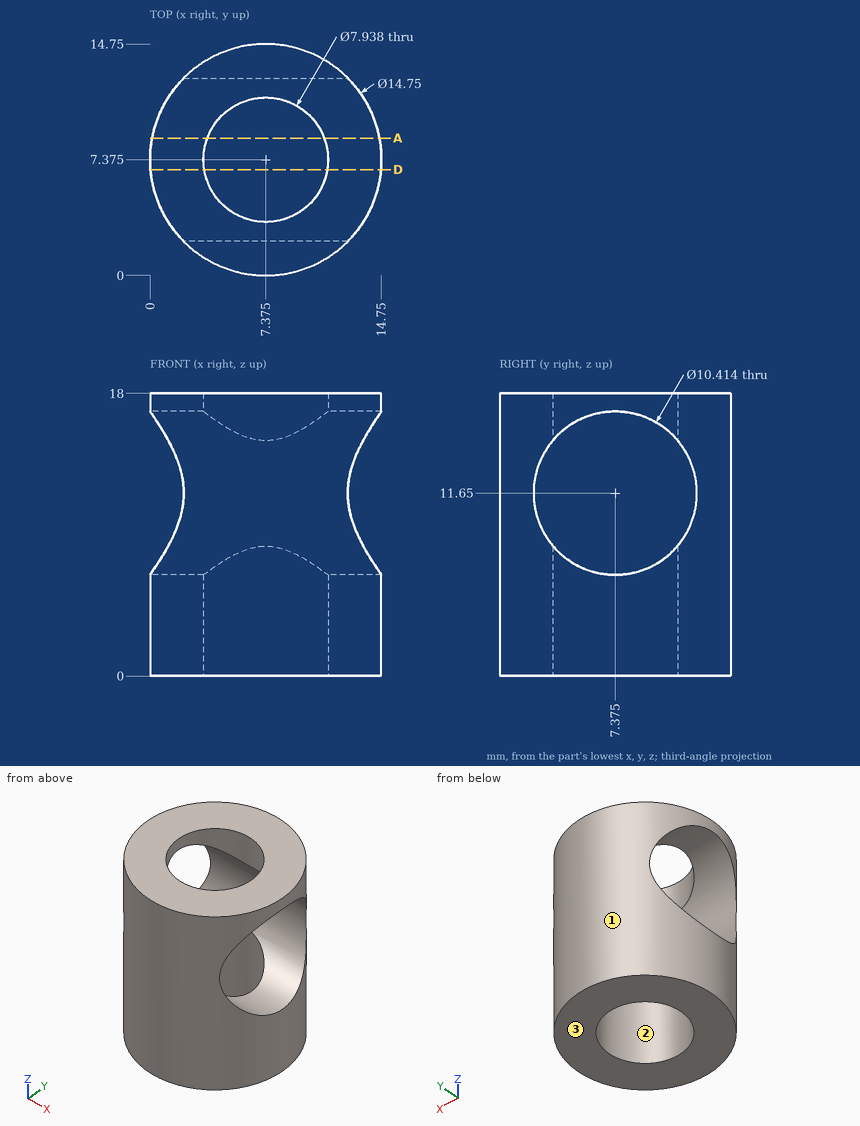
Geometry: see drawing. Coordinates: mm, zero at the bounding-box minimum. Give positions to 0.01 mm unless a question says otherwise; leave off trailing zeros. Order: outer loops, then holes, each group sorted by start corner. A loop starts at its lowest first (then second) coordinate and runs counter-clockwise, first axis right, second up. Notation, with made-up numbers: (6.25, 78) -> (52.25, 78) arc R20 cw to (52.25, 100) -> close; hole circle Ø9 at (-24.5, 16). An arc over 180 degrees is marked (long way). Write each question's results on one line, items separated by ' | '. Start each with the question number.
1) Line query: line 1 (Z direction, x = 1, y = 7.5) (1 decimal); line 2 (Y direction, x = 11.75, z = 16.25) (1 decimal); line 3 (Z direction, x = 11.5, y = 3) (1 decimal). Output: solid intervals per line, ascending. Write a range as from..to.
2) Draft query along Y for the marked faces 1, 2 and 3. Return one class per face: pulls with the +Y half, pulls with the -Y half, needs draft (parallel to the pull), parting line crosses it, or undercut.
3) Section A-A (y = 8.75). Return loops of the section in (x, z).
4) Section D-D (y = 6.75). Return loops of the section in (x, z) (1 decimal).
5) First-contact query: pin 1 (1 mm diameter, centred on y = 3, z = 15.5, fed in from -X); pin 2 (1 mm diameter, centred on y = 11.5, z = 8, fed in from +X) (1 decimal); pin 3 (2 mm diameter, centred on x = 12, z = 4.5, fed in from -Y). Flat tips, straight axial feed; report the tip coordinate or a pass-through.
Calculated:
1) line 1: 0..6.4, 16.9..18 | line 2: 1.4..4.9, 9.8..13.3 | line 3: 0..8.8, 14.5..18
2) face 1: parting line crosses it | face 2: undercut | face 3: needs draft
3) outline: (0.13, 0) -> (3.65, 0) -> (3.65, 6.63) -> (0.13, 6.63) -> close; (0.13, 16.67) -> (3.65, 16.67) -> (3.65, 18) -> (0.13, 18) -> close; (11.1, 0) -> (14.62, 0) -> (14.62, 6.63) -> (11.1, 6.63) -> close; (11.1, 16.67) -> (14.62, 16.67) -> (14.62, 18) -> (11.1, 18) -> close
4) outline: (0, 0) -> (3.5, 0) -> (3.5, 6.5) -> (0, 6.5) -> close; (0, 16.8) -> (3.5, 16.8) -> (3.5, 18) -> (0, 18) -> close; (11.3, 0) -> (14.7, 0) -> (14.7, 6.5) -> (11.3, 6.5) -> close; (11.3, 16.8) -> (14.7, 16.8) -> (14.7, 18) -> (11.3, 18) -> close
5) pin 1: x = 1.1 | pin 2: x = 13.8 | pin 3: y = 0.95
